```python
from build123d import *

# Parameters (mm, degrees)
BOSS_EXTRUDE1_DEPTH      = 6
BOSS_EXTRUDE1_DEPTH_BACK = 6
SKETCH1_W                = 12
SKETCH1_H                = 5
SKETCH2_R                = 1
CUT_EXTRUDE1_DEPTH       = 12
SKETCH3_W                = 6
SKETCH3_H                = 5
SKETCH3_R                = 1
BOSS_EXTRUDE2_DEPTH      = 3
FILLET1_R                = 2
FILLET1_OF_MIRROR1_R     = 2


with BuildPart() as part:
    # Sketch1 → Boss-Extrude1 (new, two sides: drawn at the far end of the back side and taken through both)
    with BuildSketch(Plane.XY.offset(-BOSS_EXTRUDE1_DEPTH_BACK)):
        Rectangle(SKETCH1_W, SKETCH1_H)
    extrude(amount=BOSS_EXTRUDE1_DEPTH + BOSS_EXTRUDE1_DEPTH_BACK)

    # Sketch2 → Cut-Extrude1 (cut)
    with BuildSketch(Plane.XY.offset(6)):
        with Locations((-3, 0)):
            Circle(SKETCH2_R)
        with Locations((3, 0)):
            Circle(SKETCH2_R)
    extrude(amount=-CUT_EXTRUDE1_DEPTH, mode=Mode.SUBTRACT)

    # Sketch3 → Boss-Extrude2 (add)
    with BuildSketch(Plane(origin=(6, 0, 0), x_dir=(0, 0, -1), z_dir=(1, 0, 0))):
        with Locations((0, -5)):
            Rectangle(SKETCH3_W, SKETCH3_H)
        with Locations((0, -5)):
            Circle(SKETCH3_R, mode=Mode.SUBTRACT)
    boss_extrude2 = extrude(amount=-BOSS_EXTRUDE2_DEPTH)

    # Fillet1
    fillet1_edges = [part.edges().sort_by_distance(p)[0] for p in [
        (4.5, -7.5, 3),
        (4.5, -7.5, -3),
    ]]
    fillet(fillet1_edges, radius=FILLET1_R)

    # Mirror1: Boss-Extrude2 across plane
    add(boss_extrude2.mirror(Plane(origin=(0, 0, 0), x_dir=(0, 0, 1), z_dir=(1, 0, 0))))

    # Fillet1 of Mirror1
    fillet1_of_mirror1_edges = [part.edges().sort_by_distance(p)[0] for p in [
        (-4.5, -7.5, 3),
        (-4.5, -7.5, -3),
    ]]
    fillet(fillet1_of_mirror1_edges, radius=FILLET1_OF_MIRROR1_R)


solid = part.part
```
Geometry: final body of the model. Coordinates: model frame, mm. A direction names the side the tool comes from. Coordinates: 2 decimals unless noted, no trailing zeros. Order: outer loops, then holes, each group sorted by start corner. A loop starts at its lowest first (then second) coordinate and runs counter-clockwise, first axis right, second up. Notation, with made-up numbers: M -13.5,-6.5 L 3.5,-6.5 A21 cw 3.5,3.5 Z; hole C 56.5,15 d9. An arc over 180 degrees is marked long. Answer in a Markdown table with one row per item. Add a question column.
Q1. Section query A-A on x = 4.5. Return the cut outline in (y, z).
Q2. Line query: L1, parallel to X at y = -5.5, z = -2; L2, parallel to Y at x = -4.4, z = 0; L3, parallel to X at y = 0.5, z = -3.75. Output: solid intervals per line, ascending.
Q3. Reachability of faces 1 (the flat face through (-5, -4, 3)), 2 (the flat face through (3, -3.85, 0.04)), 3 (the flat face through (-5, -4, -3)) from +Z, -Z, +X, -X, +Y, -Y: full face, straight path, thin tool, end or side. Return the list, or none.
Q4. Section query C-C on x = -3.25. Return the cut outline in (y, z).
Q5. Section query D-D on y = -5. Return the cut outline in (x, z), and give its area (3 significant figures).
Q6. Contact query for flat-ended pins moving along their axis: P1, Ø0.9, axis at x = 4.5, y = -4.5, coming from the -Z side; P2, Ø1.6, axis at y = -5, z = 0, coming from the +X side; P3, Ø1.5, axis at x = 0, z = -0.5, coming from the -Y side; P4, Ø0.9, axis at x = -4, y = -3.5, coming from the +Z side. Output: stop coordinate, or through.
Q7. Mould query, pull axis Z, two halves, no side actions, for faces 4 (the cylindrical face through (-5, -4, 0)), 5 (the cylindrical face through (4.48, -6.9, 2.43)), 6 (the flat face through (5, -7.5, 0)). Classes: released by +Z, released by -Z, zero draft, split by the parting line, or undercut.
Q8. Section query B-B on y = -3.5. Return the cut outline in (x, z).
Completed:
| question | item | result |
|---|---|---|
| 1 | outline | M -7.5,-1 A2 ccw -5.5,-3 L -2.5,-3 L -2.5,-6 L 2.5,-6 L 2.5,6 L -2.5,6 L -2.5,3 L -5.5,3 A2 ccw -7.5,1 Z; hole C -5,0 d2 |
| 2 | L1 | x = -6 to -3, 3 to 6 |
| 2 | L2 | y = -7.5 to -6, -4 to 2.5 |
| 2 | L3 | x = -6 to -3.87, -2.13 to 2.13, 3.87 to 6 |
| 3 | face 1 | +Z, +X, -X, -Y |
| 3 | face 2 | +Z, -Z, -Y |
| 3 | face 3 | -Z, +X, -X, -Y |
| 4 | outline | M -7.5,-1 A2 ccw -5.5,-3 L -2.5,-3 L -2.5,-6 L -0.97,-6 L -0.97,6 L -2.5,6 L -2.5,3 L -5.5,3 A2 ccw -7.5,1 Z; M 0.97,-6 L 2.5,-6 L 2.5,6 L 0.97,6 Z; hole C -5,0 d2 |
| 5 | outline | M -6,-3 L -3,-3 L -3,-1 L -6,-1 Z; M -6,1 L -3,1 L -3,3 L -6,3 Z; M 3,-3 L 6,-3 L 6,-1 L 3,-1 Z; M 3,1 L 6,1 L 6,3 L 3,3 Z |
| 5 | area | 24.0 mm2 |
| 6 | P1 | stops at z = -3 |
| 6 | P2 | passes through |
| 6 | P3 | stops at y = -2.5 |
| 6 | P4 | stops at z = 3 |
| 7 | face 4 | undercut |
| 7 | face 5 | released by +Z |
| 7 | face 6 | zero draft |
| 8 | outline | M -6,-3 L -3,-3 L -3,3 L -6,3 Z; M 3,-3 L 6,-3 L 6,3 L 3,3 Z |
